Geometry check sheet. Reference: the model listing, model coordinates, mm. A direction names the side the tool comes from. Round coordinates to 2 decimals unless told otherwise and drop trailing zeros. Write each loop counter-clockwise with the first axis right and the second up, starting at its lowest first coordinate (ties: lowest second). Pieces come first, ordered by that corner, then holes. Notation, with made-up numbers: (57, 28) - (84, 28) arc R29 ccw to (84, 54) - close; hole circle Ø10 at (72.25, -40). An arc over 180 degrees is marked (long way). Return JSON: item names as keys, results as strings.
```python
from build123d import *

# Parameters (mm, degrees)
BOSS_EXTRUDE1_DEPTH = 2.794
SKETCH2_W           = 3.302
SKETCH2_H           = 5.715
CUT_EXTRUDE1_DEPTH  = 53.731311505


with BuildPart() as part:
    # Sketch1 → Boss-Extrude1 (new, symmetric)
    with BuildSketch(Plane.XY):
        Polygon((-19.05, -27.813), (-19.05, -22.225), (-2.38125, -22.225), (-2.38125, -16.66875), (-4.7625, -16.66875), (-4.7625, -11.90625), (-2.38125, -11.90625), (-2.38125, -6.35), (2.38125, -6.35), (2.38125, -11.90625), (4.7625, -11.90625), (4.7625, -16.66875), (2.38125, -16.66875), (2.38125, -22.225), (19.05, -22.225), (19.05, -27.813), (44.45, -27.813), (44.45, -22.225), (44.45, 22.225), (44.45, 27.813), (19.05, 27.813), (19.05, 22.225), (2.38125, 22.225), (2.38125, 16.66875), (4.7625, 16.66875), (4.7625, 11.90625), (2.38125, 11.90625), (2.38125, 6.35), (-2.38125, 6.35), (-2.38125, 11.90625), (-4.7625, 11.90625), (-4.7625, 16.66875), (-2.38125, 16.66875), (-2.38125, 22.225), (-19.05, 22.225), (-19.05, 27.813), (-44.45, 27.813), (-44.45, 22.225), (-44.45, -22.225), (-44.45, -27.813), align=None)
    extrude(amount=BOSS_EXTRUDE1_DEPTH, both=True)

    # Sketch2 → Cut-Extrude1 (cut, through all)
    with BuildSketch(Plane.XY.offset(2.794)):
        with Locations((-38.675056, -9.11225)):
            Rectangle(SKETCH2_W, SKETCH2_H)
        with Locations((38.675056, -9.11225)):
            Rectangle(SKETCH2_W, SKETCH2_H)
    extrude(amount=-CUT_EXTRUDE1_DEPTH, mode=Mode.SUBTRACT)


solid = part.part
```
(1) Release check for a two-part mould opening along Y. For faces 1 (the face through (39, -11.97, 0)), 2 (the face through (11, 22.225, 0)), 3 (the face through (-4, 11.906, 0)), 4 (the face through (-1, 0, -2.794)) record: pulls with the +Y half, pulls with the -Y half, needs draft (parallel to the pull), parting line crosses it, or undercut.
Response values:
{"face 1": "undercut", "face 2": "pulls with the +Y half", "face 3": "undercut", "face 4": "needs draft"}
(2) Section check A-A, the plane y = -21. Enter the section's corners in (x, z).
Response values:
{"outline": "(-44.45, -2.79) - (-2.38, -2.79) - (-2.38, 2.79) - (-44.45, 2.79) - close; (2.38, -2.79) - (44.45, -2.79) - (44.45, 2.79) - (2.38, 2.79) - close"}
(3) Section check C-C, the plane x = -7. Enter the section's corners in (y, z) (3 decimals), plus the area to 3 significant figures.
Response values:
{"outline": "(-22.225, -2.794) - (22.225, -2.794) - (22.225, 2.794) - (-22.225, 2.794) - close", "area": "248 mm^2"}
(4) Material ranges on line 1 along X through (y, z) = (16.5, -0.05); line 2 along X through (y, z) = (9.5, -1.55); line 3 along X through (y, z) = (-10.5, 2), recorded low to high. Write a range as [from, to].
Response values:
{"line 1": "x = [-44.45, -4.76], [4.76, 44.45]", "line 2": "x = [-44.45, -2.38], [2.38, 44.45]", "line 3": "x = [-44.45, -40.33], [-37.02, -2.38], [2.38, 37.02], [40.33, 44.45]"}
(5) Section check B-B, the plane y = -8. Enter the section's corners in (x, z), plus the area to 3 significant figures.
Response values:
{"outline": "(-44.45, -2.79) - (-40.33, -2.79) - (-40.33, 2.79) - (-44.45, 2.79) - close; (-37.02, -2.79) - (-2.38, -2.79) - (-2.38, 2.79) - (-37.02, 2.79) - close; (2.38, -2.79) - (37.02, -2.79) - (37.02, 2.79) - (2.38, 2.79) - close; (40.33, -2.79) - (44.45, -2.79) - (44.45, 2.79) - (40.33, 2.79) - close", "area": "433 mm^2"}
(6) Access from +Z, -Z, +X, -X, +Y, -Y to the whole of each face (thin tool, end or side, straight path). Record for faces 5 (the face through (2.381, -9, 0)), 6 (the face through (4.762, -14, 0)), 7 (the face through (44.45, 0, 0)), 8 (the face through (0, 6.35, 0)).
Response values:
{"face 5": "+Z, -Z, -Y", "face 6": "+Z, -Z", "face 7": "+Z, -Z, +X, +Y, -Y", "face 8": "+Z, -Z, +Y"}
(7) Section check D-D, the plane z = -0.2. Give the number of separate pieces and of enclosed holes in the cut face, plus the area to 3 significant figures.
Response values:
{"separate pieces": "1", "enclosed holes": "2", "area": "4,290 mm^2"}
(8) Gauge pin test, flat ends, axial feed: pin 1 (1.9 mm diameter, centred on x = -3.5, z = -1, fed in from -Y) (3 decimals); pin 2 (1.9 mm diameter, centred on x = 3, z = -1.5, fed in from +Y) (3 decimals); pin 3 (1.4 mm diameter, centred on x = -0.5, z = 1, fed in from -Y). Record the tip position at first contact, or that the pin passes through.
Response values:
{"pin 1": "stops at y = -22.225", "pin 2": "stops at y = 22.225", "pin 3": "stops at y = -6.35"}
